Geometry: final body of the model. Coordinates: model frame, mm. A direction names the side the tool comes from. Coordinates: 2 decimals unless noted, no trailing zeros. Write each loop counter-clockwise with the first axis right and the second up, starting at its lowest first coordinate (ties: lowest second). Pieces come first, ordered by that corner, then holes. Notation, with made-up numbers: (-34.5, -10.5) -> (9.5, -10.5) arc R26 ccw to (9.5, 27.5) -> close; hole circle Ø11 at (70, 37). An arc over 180 degrees is marked (long way). One line per item, written item: value. Start each with the question number.
Autodesk Inventor part; units mm, degrees
ref_plane "YZ Plane" through (0, 0, 0) normal (1, 0, 0) x (0, 1, 0)
ref_plane "XZ Plane" through (0, 0, 0) normal (0, 1, 0) x (-1, 0, 0)
ref_plane "XY Plane" through (0, 0, 0) normal (0, 0, 1) x (1, 0, 0)
sketch "Skizze1" plane through (0, 0, 0) normal (0, 0, 1) x (1, 0, 0)
  line L0 (0, 0) -> (23, 0)
  line L1 (23, 0) -> (23, -31)
  line L2 (23, -31) -> (0, -31)
  line L3 (0, -31) -> (0, 0)
  line L4 (2.56, -2.75) -> (20.44, -2.75) construction
  line L5 (20.44, -2.75) -> (20.44, -28.25) construction
  line L6 (20.44, -28.25) -> (2.56, -28.25) construction
  line L7 (2.56, -28.25) -> (2.56, -2.75) construction
  circle A0 centre (2.56, -2.75) radius 1.5
  circle A1 centre (20.44, -2.75) radius 1.5
  circle A2 centre (2.56, -28.25) radius 1.5
  circle A3 centre (20.44, -28.25) radius 1.5
  line L8 (4.56, -4.75) -> (18.44, -4.75)
  line L9 (18.44, -4.75) -> (18.44, -26.25)
  line L10 (18.44, -26.25) -> (4.56, -26.25)
  line L11 (4.56, -26.25) -> (4.56, -4.75)
  dimension "d0" = 23
  dimension "d1" = 31
  dimension "d2" = 17.88
  dimension "d3" = 25.5
  dimension "d4" = 2.75
  dimension "d5" = 2.56
  dimension "d6" = 3
  dimension "d7" = 3
  dimension "d8" = 3
  dimension "d9" = 3
  dimension "d10" = 2
  dimension "d11" = 2
  dimension "d12" = 2
  dimension "d13" = 2
extrude "Extrusion1" add sketch "Skizze1" along normal blind 3
sketch "Skizze2" plane through (0, 0, 3) normal (0, 0, 1) x (1, 0, 0)
  line L0 (5.1, -31) -> (17.9, -31)
  line L1 (17.9, -31) -> (17.9, -27.6)
  line L2 (17.9, -27.6) -> (5.1, -27.6)
  line L3 (5.1, -27.6) -> (5.1, -31)
  line L4 (23, 0) -> (0, 0)
  line L5 (5.1, 0) -> (17.9, 0)
  line L6 (17.9, 0) -> (17.9, -3.4)
  line L7 (17.9, -3.4) -> (5.1, -3.4)
  line L8 (5.1, -3.4) -> (5.1, 0)
  line L9 (0, -31) -> (23, -31)
  line L10 (0, 0) -> (0, -31)
  dimension "d16" = 3.4
  dimension "d17" = 3.4
  dimension "d18" = 12.8
  dimension "d19" = 5.1
extrude "Extrusion2" cut sketch "Skizze2" against normal blind 3
chamfer "Fase1" distance 2 angle 45 4 edges at (4.56, -4.75, 1.5) (18.44, -4.75, 1.5) (4.56, -26.25, 1.5) (18.44, -26.25, 1.5)
properties part number "CFV4_Scale_HX711_Baseplate" material "ABS-Kunststoff"
Q1. Cut plane B-B on x = 2.56. Output: boundary loops of the cut face in (y, z), and give its area (3 significant figures).
Q2. Cut plane D-D on x = 13. Output: boundary loops of the cut face in (y, z).
Q3. Cut plane C-C on z = 2. Output: boundary loops of the cut face in (x, y).
Q4. Line query: L1, parallel to Y at x = 2.56, z = 1.7; L2, parallel to X at y = -21, z = 0.9; L3, parallel to Y at x = 15.25, z = 0.6. Output: solid intervals per line, ascending. Write a range as from..to.
Q5. Access query for faces 4 (the flat face through (3, 0, 1)), 5 (the flat face through (5.1, -2, 2)), 6 (the flat face through (17.45, -5.76, 1.48)), 7 (the flat face through (12, -27.6, 2)). Directions: +Z, -Z, +X, -X, +Y, -Y. A direction counts if a zero-diameter tool reaches every point of the face in a straight line with its end or side. Return the directions, or none.
Q6. Draft query along Y for faces 1 (the flat face through (5.57, -5.74, 1.48)), 2 (the flat face through (3, -31, 1)), 3 (the flat face through (17.9, -2, 2)). Return one class per face: pulls with the +Y half, pulls with the -Y half, needs draft (parallel to the pull), parting line crosses it, or undercut.
Q7. First-contact query: P1, Ø0.9, axis at x = 9.5, z = 1, coming from the +Y side; P2, Ø0.9, axis at x = 11.5, z = 2, coming from the -Y side; P3, Ø5, axis at x = 17, y = -26.5, coming from the -Z side. Flat tips, straight axial feed; report the tip coordinate or a pass-through.
Q8. Cut plane A-A on y = -28.25. Output: boundary loops of the cut face in (x, z).
Solution:
1. outline: (-31, 0) -> (-29.75, 0) -> (-29.75, 3) -> (-31, 3) -> close; (-26.75, 0) -> (-4.25, 0) -> (-4.25, 3) -> (-26.75, 3) -> close; (-1.25, 0) -> (0, 0) -> (0, 3) -> (-1.25, 3) -> close
1. area: 75.0 mm²
2. outline: (-27.6, 0) -> (-26.25, 0) -> (-26.25, 3) -> (-27.6, 3) -> close; (-4.75, 0) -> (-3.4, 0) -> (-3.4, 3) -> (-4.75, 3) -> close
3. outline: (0, -31) -> (5.1, -31) -> (5.1, -27.6) -> (17.9, -27.6) -> (17.9, -31) -> (23, -31) -> (23, 0) -> (17.9, 0) -> (17.9, -3.4) -> (5.1, -3.4) -> (5.1, 0) -> (0, 0) -> close; hole circle Ø3 at (2.56, -28.25); hole circle Ø3 at (2.56, -2.75); hole (4.56, -24.25) -> (6.56, -26.25) -> (16.44, -26.25) -> (18.44, -24.25) -> (18.44, -6.75) -> (16.44, -4.75) -> (6.56, -4.75) -> (4.56, -6.75) -> close; hole circle Ø3 at (20.44, -28.25); hole circle Ø3 at (20.44, -2.75)
4. L1: -31..-29.75, -26.75..-4.25, -1.25..0
4. L2: 0..4.56, 18.44..23
4. L3: -27.6..-26.25, -4.75..-3.4
5. face 4: +Z, -Z, +X, -X, +Y
5. face 5: +Z, -Z, +Y
5. face 6: +Z, -Z
5. face 7: +Z, -Z, -Y
6. face 1: undercut
6. face 2: pulls with the -Y half
6. face 3: needs draft
7. P1: y = -3.4
7. P2: y = -27.6
7. P3: z = 0
8. outline: (0, 0) -> (1.06, 0) -> (1.06, 3) -> (0, 3) -> close; (4.06, 0) -> (5.1, 0) -> (5.1, 3) -> (4.06, 3) -> close; (17.9, 0) -> (18.94, 0) -> (18.94, 3) -> (17.9, 3) -> close; (21.94, 0) -> (23, 0) -> (23, 3) -> (21.94, 3) -> close
